```python
from build123d import *

# Parameters (mm, degrees)
F0_W     = 58.674
F0_H     = 59.69
F0_R     = 1.524
F0_W_2   = 12.7
F0_H_2   = 11.43
F0_R_2   = 1.651
F0_W_3   = 27.178
F0_H_3   = 10.16
F1_DEPTH = 1.27
F2_W     = 58.674
F2_H     = 59.69
F2_W_2   = 39.878
F2_H_2   = 15.24
F2_W_3   = 40.64
F2_H_3   = 13.97
F3_DEPTH = 1.27
F4_R     = 6.35
F5_R     = 1.27
F6_R     = 1.905
F7_DEPTH = 2.54


with BuildPart() as f1:
    # F0 (on Top) → F1 (new body)
    with BuildSketch(Plane.XY):
        with Locations((0, -12.065)):
            Rectangle(F0_W, F0_H)
        with Locations((-12.954, -23.495)):
            Circle(F0_R, mode=Mode.SUBTRACT)
        with Locations((0, -23.495)):
            Rectangle(F0_W_2, F0_H_2, mode=Mode.SUBTRACT)
        with Locations((12.954, -23.495)):
            Circle(F0_R, mode=Mode.SUBTRACT)
        with Locations((-16.637, 0)):
            Circle(F0_R_2, mode=Mode.SUBTRACT)
        Rectangle(F0_W_3, F0_H_3, mode=Mode.SUBTRACT)
        with Locations((16.637, 0)):
            Circle(F0_R_2, mode=Mode.SUBTRACT)
    extrude(amount=F1_DEPTH)

    # F2 (on face) → F3 (join)
    with BuildSketch(Plane.XY.offset(1.27)):
        with Locations((0, -12.065)):
            Rectangle(F2_W, F2_H)
        with Locations((0, -23.495)):
            Rectangle(F2_W_2, F2_H_2, mode=Mode.SUBTRACT)
        Rectangle(F2_W_3, F2_H_3, mode=Mode.SUBTRACT)
    extrude(amount=F3_DEPTH)

    # F4
    f4_edges = [f1.edges().sort_by_distance(p)[0] for p in [
        (-29.337, -41.91, 1.27),
        (29.337, 17.78, 1.27),
        (29.337, -41.91, 1.27),
        (-29.337, 17.78, 1.27),
    ]]
    fillet(f4_edges, radius=F4_R)

    # F5
    f5_edges = [f1.edges().sort_by_distance(p)[0] for p in [
        (-27.477128, -40.050128, 0),
        (-13.589, 5.08, 0.635),
        (-13.589, -5.08, 0.635),
        (13.589, -5.08, 0.635),
        (13.589, 5.08, 0.635),
    ]]
    fillet(f5_edges, radius=F5_R)

    # F6 (on face) → F7 (cut, through all)
    with BuildSketch(Plane.XY.offset(2.54)):
        with Locations((-22.987, 11.43)):
            Circle(F6_R)
        with Locations((22.987, 11.43)):
            Circle(F6_R)
        with Locations((22.987, -35.56)):
            Circle(F6_R)
        with Locations((-22.987, -35.56)):
            Circle(F6_R)
    extrude(amount=-F7_DEPTH, mode=Mode.SUBTRACT)


solid = f1.part
```
Design review of the part built by this model. Coordinates are the model's own, in mm. A direction names the side the tool comes from. Coordinates: 2 decimals unless noted, no trailing zeros. Write each loop counter-clockwise with the first axis right and the second up, starting at its lowest first coordinate (ties: lowest second). Pieces come first, ordered by that corner, then holes.
1) To check wall thickness, follow L1, parallel to Y at x = -5, z = 1.75 (3 decimals); L2, parallel to Y at x = -2, z = 1.1; L3, parallel to X at y = -28.5, z = 1.7. State the ranges of each line that lie inside material, in increasing order.
2) Add section A-A (x = 8). Write out the cut boundary in (y, z) (3 decimals), plus the area to 3 significant figures.
3) Add section C-C (z = 1.7). Write out the cut boundary in (x, y) (3 decimals), plus the area to 3 significant figures.
4) Insertion check: pin 1 (1 mm diameter, centred on y = -23.5, z = 0.5, fed in from -X); pin 2 (5 mm diameter, centred on x = -22.987, y = -35.56, fed in from -Z); pin 3 (0.6 mm diameter, centred on y = 2, z = 0.5, fed in from -X); pin 4 (4 mm diameter, centred on x = 17.5, y = -26.5, fed in from +Z). Each pin has a flat end and moves straight along its axis. Give the tip position at first contact, or say it passes through.
5) Mouldability with a two-part tool opening along Y and no side actions: class faces 4 (the flat face through (-19.939, -24, 2)), 5 (the cylindrical face through (27.427, -40.099, 1.914)), 6 (the flat face through (29.337, -12, 2)) as +Y half, -Y half, draft (parallel to the pull), parting line (faces both ways), or undercut.
6) Machinability: for faces 1 (the flat face through (0, -12, 0)), 2 (the cylindrical face through (-13.207, -4.718, 0.644)), 3 (the flat face through (0, -17, 1.27)), which of the approach directions +Z, -Z, +X, -X, +Y, -Y give a long, thin tool a straight path to every point of the face, cutting with its end or side? Answer none if there is none.
7) Add section B-B (y = 0). Write out the cut boundary in (x, z), plus the area to 3 significant figures.
Check result:
1. L1: y = -41.91 to -31.115, -15.875 to -6.985, 6.985 to 17.78
1. L2: y = -41.9 to -29.21, -17.78 to -5.08, 5.08 to 17.77
1. L3: x = -29.34 to -19.94, 19.94 to 29.34
2. outline: (-41.91, 1.27) arc R1.27 ccw to (-40.64, 0) - (-5.08, 0) - (-5.08, 1.27) - (-6.985, 1.27) - (-6.985, 2.54) - (-15.875, 2.54) - (-15.875, 1.27) - (-31.115, 1.27) - (-31.115, 2.54) - (-41.91, 2.54) - close; (5.08, 0) - (16.51, 0) arc R1.27 ccw to (17.78, 1.27) - (17.78, 2.54) - (6.985, 2.54) - (6.985, 1.27) - (5.08, 1.27) - close
2. area: 101 mm2
3. outline: (-29.337, -35.56) arc R6.35 ccw to (-22.987, -41.91) - (22.987, -41.91) arc R6.35 ccw to (29.337, -35.56) - (29.337, 11.43) arc R6.35 ccw to (22.987, 17.78) - (-22.987, 17.78) arc R6.35 ccw to (-29.337, 11.43) - close; hole circle Ø3.81 at (-22.987, -35.56); hole circle Ø3.81 at (-22.987, 11.43); hole (-20.32, -6.985) - (20.32, -6.985) - (20.32, 6.985) - (-20.32, 6.985) - close; hole (-19.939, -31.115) - (19.939, -31.115) - (19.939, -15.875) - (-19.939, -15.875) - close; hole circle Ø3.81 at (22.987, -35.56); hole circle Ø3.81 at (22.987, 11.43)
3. area: 2,250 mm2
4. pin 1: stops at x = -29.31
4. pin 2: stops at z = 0
4. pin 3: stops at x = -29.25
4. pin 4: stops at z = 1.27
5. face 4: undercut
5. face 5: -Y half
5. face 6: draft
6. face 1: -Z, +X, -X, +Y, -Y
6. face 2: +Z, -Z
6. face 3: +Z
7. outline: (-29.34, 1.27) arc R1.27 ccw to (-28.07, 0) - (-18.29, 0) - (-18.29, 1.27) - (-20.32, 1.27) - (-20.32, 2.54) - (-29.34, 2.54) - close; (-14.99, 0) - (-13.59, 0) - (-13.59, 1.27) - (-14.99, 1.27) - close; (13.59, 0) - (14.99, 0) - (14.99, 1.27) - (13.59, 1.27) - close; (18.29, 0) - (28.07, 0) arc R1.27 ccw to (29.34, 1.27) - (29.34, 2.54) - (20.32, 2.54) - (20.32, 1.27) - (18.29, 1.27) - close
7. area: 53.8 mm2
